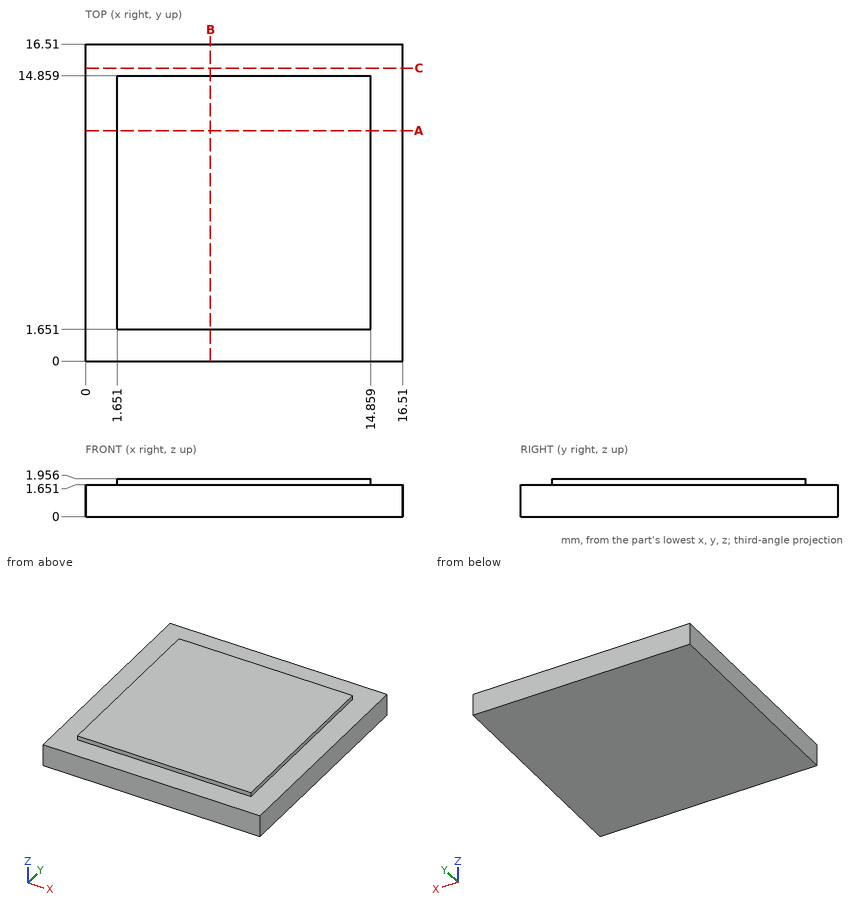
The drawing under review shows one solid part. Ordinate dimensions are in mm from its lowest x, y, z. Give positions to 0.01 mm unless a question says otherwise; leave off trailing zeros. Loops run counter-clockwise (first coordinate to the right, second up) from the corner with the lowest first, then second, coordinate; pieces in that order, holes last. Notation, with made-up numbers: M -4,68 L 52,68 A21 ccw 52,99 Z; hole C -13,64.25 d10. An arc over 180 degrees is marked long. One line per question, with ' | ' between items. Start each with the question number.
1. Add section A-A (y = 12). Write out the cut boundary in (x, z), plus the area to 3 significant figures.
2. Add section C-C (y = 15.25). Write out the cut boundary in (x, z).
3. Insertion check: P1, Ø3, axis at x = 3, y = 11, coming from the -Z side. The pin has a flat end and moves straight along its axis. Give the tip position at first contact, or say it passes through.
4. To check wall thickness, follow L1, parallel to X at y = 10.5, z = 1.75; L2, parallel to Z at x = 1.5, y = 2.75. State the ranges of each line that lie inside material, in increasing order.
Worked out:
1) outline: M 0,0 L 16.51,0 L 16.51,1.65 L 14.86,1.65 L 14.86,1.96 L 1.65,1.96 L 1.65,1.65 L 0,1.65 Z | area: 31.3 mm²
2) outline: M 0,0 L 16.51,0 L 16.51,1.65 L 0,1.65 Z
3) P1: stops at z = 0
4) L1: x = 1.65 to 14.86 | L2: z = 0 to 1.65
